Answer from the drawing. Dimensions are ordinates in mm from the lowest x, y and z of the part. A direction names the side the tool comes from. Coordinates: 2 decimals unless noted, no trailing zeros. Order: outer loops, then holes, each group sorted by start corner. A loop starts at its lowest first (then second) coordinate and runs counter-clockwise, first axis right, second up. Notation, with made-up numbers: (70, 56) -> (76, 56) arc R21 ccw to (76, 91) -> close; hole circle Ø4 at (-2.75, 65.25). An arc over 180 degrees is marked (long way). Answer in a Markdown table with one row per item.
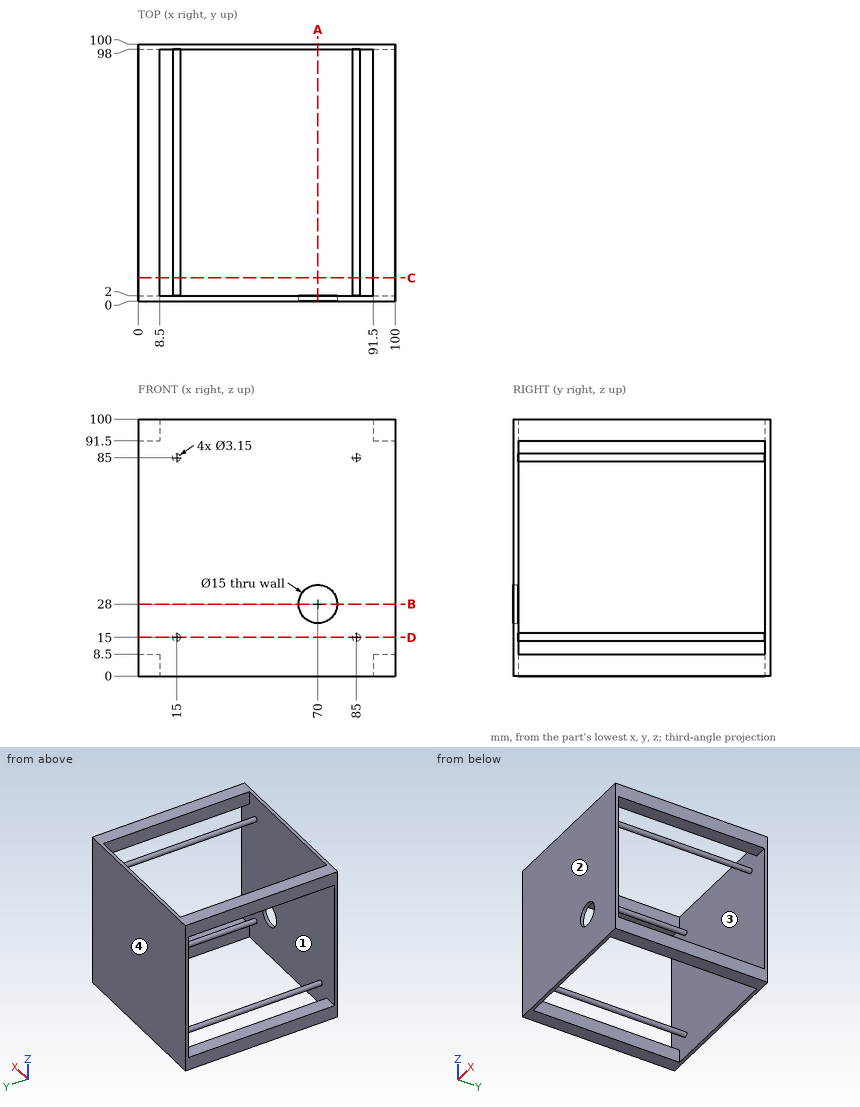
(1) Which of the six approach directions +Z, -Z, +X, -X, +Y, -Y give full straight-line access (tool end or side, diameter ignored) to the marked faces 3 and 4?
Check values:
| item | result |
|---|---|
| face 3 | none |
| face 4 | +Z, -Z, +X, -X, +Y |
(2) A cutting plane is placed at B-B, the plane z = 28. Determine the outline of the cut face in (x, y), then the cut area to 3 significant figures.
Check values:
| item | result |
|---|---|
| outline | (0, 0) -> (62.5, 0) -> (62.5, 2) -> (0, 2) -> close; (0, 98) -> (100, 98) -> (100, 100) -> (0, 100) -> close; (77.5, 0) -> (100, 0) -> (100, 2) -> (77.5, 2) -> close |
| area | 370 mm² |
(3) For a pull along Z with two mould halves and no side action, classify the marked faces 1 and 2 as released by +Z, released by -Z, zero draft, split by the parting line, or undercut.
Check values:
| item | result |
|---|---|
| face 1 | undercut |
| face 2 | zero draft |
(4) Flat-ended cylindrical pins translate along their axes: pin 1 (6 mm diameter, centred on x = 17, y = 27, fed in from -Z) (3 decimals); pin 2 (12 mm diameter, centred on x = 24, y = 23.5, fed in from +Z). Find the tip coordinate at first contact, or state that the pin passes through.
Check values:
| item | result |
|---|---|
| pin 1 | z = 13.425 |
| pin 2 | through |
(5) A cutting plane is placed at A-A, the plane x = 70. Determine the outline of the cut face in (y, z).
Check values:
| item | result |
|---|---|
| outline | (0, 0) -> (2, 0) -> (2, 20.5) -> (0, 20.5) -> close; (0, 35.5) -> (2, 35.5) -> (2, 100) -> (0, 100) -> close; (98, 0) -> (100, 0) -> (100, 100) -> (98, 100) -> close |
(6) A cutting plane is placed at D-D, the plane z = 15. Determine the outline of the cut face in (x, y) (3 decimals), then the cut area to 3 significant figures.
Check values:
| item | result |
|---|---|
| outline | (0, 0) -> (100, 0) -> (100, 2) -> (86.575, 2) -> (86.575, 98) -> (100, 98) -> (100, 100) -> (0, 100) -> (0, 98) -> (13.425, 98) -> (13.425, 2) -> (0, 2) -> close; hole (16.575, 2) -> (83.425, 2) -> (83.425, 98) -> (16.575, 98) -> close |
| area | 1,000 mm² |
(7) Find the intervals of material crossed by line 1 along Z through (x, y) = (15, 15.5) (3 decimals); line 2 along Y through (x, z) = (79.5, 59); line 3 along Z through (x, y) = (70, 1), in increasing order. Write a range as from..to.
Check values:
| item | result |
|---|---|
| line 1 | 13.425..16.575, 83.425..86.575 |
| line 2 | 0..2, 98..100 |
| line 3 | 0..20.5, 35.5..100 |
(8) A cutting plane is placed at C-C, the plane y = 9. Determine the outline of the cut face in (x, z) (3 decimals).
Check values:
| item | result |
|---|---|
| outline | (0, 0) -> (8.5, 0) -> (8.5, 8.5) -> (0, 8.5) -> close; (0, 91.5) -> (8.5, 91.5) -> (8.5, 100) -> (0, 100) -> close; circle Ø3.15 at (15, 15); circle Ø3.15 at (15, 85); circle Ø3.15 at (85, 15); circle Ø3.15 at (85, 85); (91.5, 0) -> (100, 0) -> (100, 8.5) -> (91.5, 8.5) -> close; (91.5, 91.5) -> (100, 91.5) -> (100, 100) -> (91.5, 100) -> close |
